Can you work these out from the model? Positions are in its coordinate system, mm. Face numbers are marked on the shaded views. A direction names the side the tool comes from. Give positions to 0.01 mm unless a question says otherwise; leave off trailing zeros. Order: outer loops, then holes, each group sorted by start corner. A loop starts at its lowest first (then second) coordinate and runs counter-clockwise, first axis right, second up. Notation, with made-up numbers: (22, 64.25) - (51, 64.25) arc R20 cw to (51, 101.25) - close; hole circle Ø8 at (54.25, -27.5). An arc over 180 degrees is marked (long way). Write each question's results on one line, items separated by ' | '. Start each with the question number.
from build123d import *

# Parameters (mm, degrees)
BOX006_W                           = 20
BOX006_H                           = 120
BOX006_DEPTH                       = 25
BOX006_PLACEMENT_ANGLE             = 5
BOX002_W                           = 20
BOX002_H                           = 57
BOX002_DEPTH                       = 17
FILLET005002_R                     = 2
BOX008_W                           = 20
BOX008_H                           = 120
BOX008_DEPTH                       = 25
BOX008_PLACEMENT_ANGLE             = 5
BOX007_W                           = 20
BOX007_H                           = 57
BOX007_DEPTH                       = 17
FILLET003001002002_R               = 2
CYLINDER_R                         = 15
CYLINDER_DEPTH                     = 120
BOX005_W                           = 20
BOX005_H                           = 120
BOX005_DEPTH                       = 25
BOX005_PLACEMENT_ANGLE             = 5
BOX004_W                           = 20
BOX004_H                           = 120
BOX004_DEPTH                       = 17
FILLET003001002003_R               = 1
FILLET003001002004_R               = 1
FILLET003001002004_PLACEMENT_ANGLE = 90


with BuildPart() as cube006:
    # Box006 → Box006 (new body)
    with BuildSketch(Plane.XY):
        with Locations((10, 60)):
            Rectangle(BOX006_W, BOX006_H)
    extrude(amount=BOX006_DEPTH)


with BuildPart() as cube006_1:
    # Box006 placement: moved
    add(cube006.part.moved(Location((-20, -60, 0))).rotate(Axis((-20, -60, 0), (0, 1, 0)), BOX006_PLACEMENT_ANGLE))


with BuildPart() as cutout002:
    # Box002 → Box002 (new body)
    with BuildSketch(Plane(origin=(0, -58.5, 0), x_dir=(1, 0, 0), z_dir=(0, 0, 1))):
        with Locations((10, 28.5)):
            Rectangle(BOX002_W, BOX002_H)
    extrude(amount=BOX002_DEPTH)

    # Cut002: cut Cube006
    add(cube006_1.part, mode=Mode.SUBTRACT)

    # Fillet005002
    fillet005002_edges = [cutout002.edges().sort_by_distance(p)[0] for p in [
        (0.076397, -30, 0),
    ]]
    fillet(fillet005002_edges, radius=FILLET005002_R)


with BuildPart() as cutout002_1:
    # Fillet005002 placement: moved
    add(cutout002.part.moved(Location((2, 0.5, 2))))


with BuildPart() as cube008:
    # Box008 → Box008 (new body)
    with BuildSketch(Plane.XY):
        with Locations((10, 60)):
            Rectangle(BOX008_W, BOX008_H)
    extrude(amount=BOX008_DEPTH)


with BuildPart() as cube008_1:
    # Box008 placement: moved
    add(cube008.part.moved(Location((-20, -60, 0))).rotate(Axis((-20, -60, 0), (0, 1, 0)), BOX008_PLACEMENT_ANGLE))


with BuildPart() as fusion:
    # Box007 → Box007 (new body)
    with BuildSketch(Plane(origin=(0, -58.5, 0), x_dir=(1, 0, 0), z_dir=(0, 0, 1))):
        with Locations((10, 28.5)):
            Rectangle(BOX007_W, BOX007_H)
    extrude(amount=BOX007_DEPTH)

    # Cut005: cut Cube008
    add(cube008_1.part, mode=Mode.SUBTRACT)

    # Fillet003001002002
    fillet003001002002_edges = [fusion.edges().sort_by_distance(p)[0] for p in [
        (0.076397, -30, 0),
    ]]
    fillet(fillet003001002002_edges, radius=FILLET003001002002_R)


with BuildPart() as fusion_1:
    # Fillet003001002002 placement: moved
    add(fusion.part.moved(Location((2, 59.5, 2))))

    # Fusion: union Cutout002
    add(cutout002_1.part)


with BuildPart() as cylinder:
    # Cylinder → Cylinder (new body)
    with BuildSketch(Plane(origin=(18.5, 60, 17), x_dir=(1, 0, 0), z_dir=(0, -1, 0))):
        Circle(CYLINDER_R)
    extrude(amount=CYLINDER_DEPTH)


with BuildPart() as cube005:
    # Box005 → Box005 (new body)
    with BuildSketch(Plane.XY):
        with Locations((10, 60)):
            Rectangle(BOX005_W, BOX005_H)
    extrude(amount=BOX005_DEPTH)


with BuildPart() as cube005_1:
    # Box005 placement: moved
    add(cube005.part.moved(Location((-20, -60, 0))).rotate(Axis((-20, -60, 0), (0, 1, 0)), BOX005_PLACEMENT_ANGLE))


with BuildPart() as fillet003001002004:
    # Box004 → Box004 (new body)
    with BuildSketch(Plane(origin=(0, -60, 0), x_dir=(1, 0, 0), z_dir=(0, 0, 1))):
        with Locations((10, 60)):
            Rectangle(BOX004_W, BOX004_H)
    extrude(amount=BOX004_DEPTH)

    # Cut003: cut Cube005
    add(cube005_1.part, mode=Mode.SUBTRACT)

    # Cut004: cut Cylinder
    add(cylinder.part, mode=Mode.SUBTRACT)

    # Cut006: cut Fusion
    add(fusion_1.part, mode=Mode.SUBTRACT)

    # Fillet003001002003
    fillet003001002003_edges = [fillet003001002004.edges().sort_by_distance(p)[0] for p in [
        (3.388727, 29.5, 17),
        (3.388727, -29.5, 17),
    ]]
    fillet(fillet003001002003_edges, radius=FILLET003001002003_R)

    # Fillet003001002004
    fillet003001002004_edges = [fillet003001002004.edges().sort_by_distance(p)[0] for p in [
        (3.5, 59, 17),
        (3.5, -59, 17),
        (3.5, 0, 17),
    ]]
    fillet(fillet003001002004_edges, radius=FILLET003001002004_R)


with BuildPart() as fillet003001002004_1:
    # Fillet003001002004 placement: moved
    add(fillet003001002004.part.rotate(Axis((0, 0, 0), (0, 0, 1)), FILLET003001002004_PLACEMENT_ANGLE))


solid = fillet003001002004_1.part
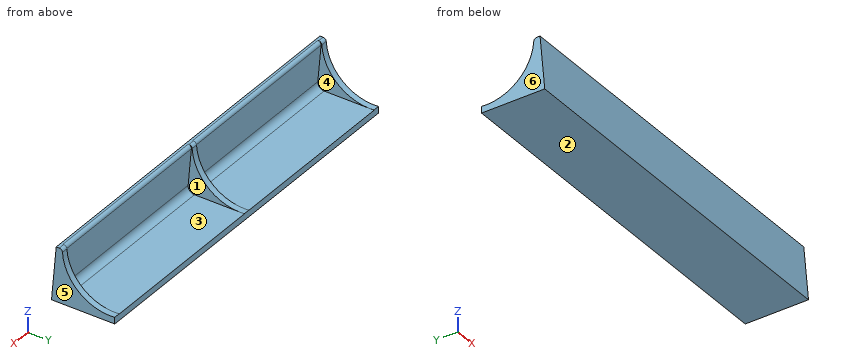
Q1. If we section it at B-B (y = 7): Please give me the cut outline in (x, z).
Q2. Will these pins go through, and if not, where does the flat tip stop? P1, Ø8, axis at x = 38.5, y = 10.5, coming from the +Z side; P2, Ø7.5, axis at y = 14.5, z = 9.5, coming from the -X side.
Q3. If I drill on probe 1 along X at (y, z) = (2.75, 3); probe 2 along Z at (x, y) = (-4.5, 14.5); probe 3 along Z at (x, y) = (-37.5, 3.5), over which ranges is the centre line in solid material (lowest first)? Write a range as from..to.
Q4. If we section it at A-A (x = 28.5): Please give me the cut outline in (y, z).
Q5. If we section it at C-C (z = 9.25): Please give me the cut outline in (x, y).
Q6. Thinking about a two-plate mould opening in X: for the marked faces 4, 5 and 6, which applies, released by +X, released by -X, zero draft, split by the parting line, or undercut?
Q7. Which directions (+Z, -Z, +X, -X, +Y, -Y) give clear straight access to the entire face, cutting with the end or side of a thin tool? Please do the marked faces 1, 2 and 3.
Findings below:
1) outline: (-60, 0) - (60, 0) - (60, 7.37) - (58, 7.37) - (58, 2) - (1, 2) - (1, 7.37) - (-1, 7.37) - (-1, 2) - (-58, 2) - (-58, 7.37) - (-60, 7.37) - close
2) P1: stops at z = 2 | P2: passes through
3) probe 1: x = -60..-58, -1..1, 58..60 | probe 2: z = 0..2 | probe 3: z = 0..2.15
4) outline: (0.08, 0) - (20, 0) - (20, 2) - (4.26, 2) arc R2 cw to (2.27, 4.17) - (3.29, 15.91) arc R1 ccw to (2.3, 17) - (1.56, 17) - close
5) outline: (-60, 0.89) - (60, 0.89) - (60, 5.66) - (58, 5.66) - (58, 2.71) - (1, 2.71) - (1, 5.66) - (-1, 5.66) - (-1, 2.71) - (-58, 2.71) - (-58, 5.66) - (-60, 5.66) - close
6) face 4: undercut | face 5: released by +X | face 6: released by -X
7) face 1: +Y | face 2: -Z, +X, -X, +Y, -Y | face 3: +Z, +Y
